Answer from the drawing. Dimensions are ordinates in mm from the lowest x, y and z of the part. Give positions to 0.01 mm unless a question says otherwise; leave off trailing zeros. Loops run counter-clockwise (first coordinate to the right, second up) from the corner with the lowest first, then second, coordinate; pieces in that order, holes last. Notation, with made-up numbers: (-0.75, 82.5) - (32.25, 82.5) arc R27 cw to (32.25, 119.5) - close; hole circle Ø2 at (47.5, 44). An arc over 180 degrees is marked (long way). One line per item, written item: value.
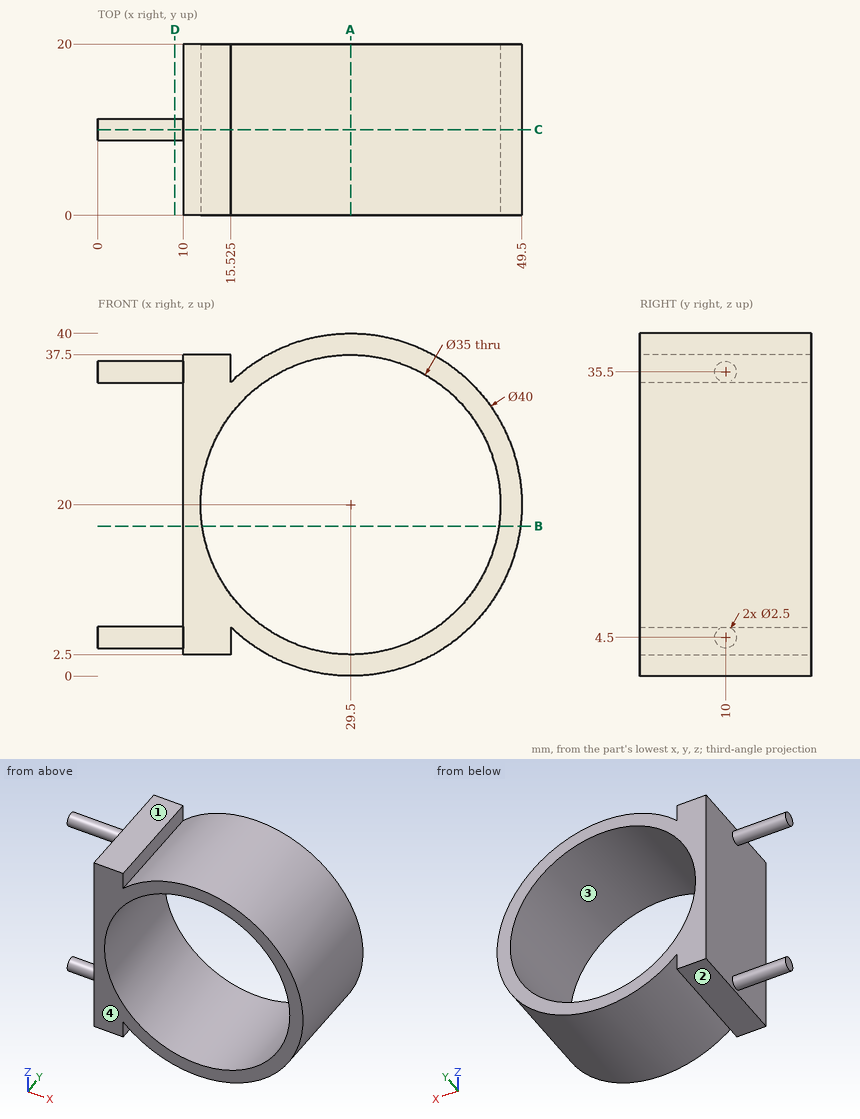
1. Flat-ended cylindrical pins translate along their axes: pin 1 Ø6 at (y, z) = (15, 11) entering from +X; pin 2 Ø3 at (x, y) = (13, 5) entering from +Z; pin 3 Ø2.5 at (y, z) = (5.5, 35.5) entering from +X; pin 4 Ø21 at (x, z) = (29.5, 20) entering from +Y. Find the tip coordinate at first contact, or state that the pin passes through.
Output:
pin 1: stops at x = 48.58
pin 2: stops at z = 37.5
pin 3: stops at x = 43.53
pin 4: passes through
2. Section A-A (x = 29.5) is taken. Write down the section's boundary in (y, z).
Output:
outline: (0, 0) - (20, 0) - (20, 2.5) - (0, 2.5) - close; (0, 37.5) - (20, 37.5) - (20, 40) - (0, 40) - close
3. Section B-B (z = 17.5) is taken. Write down the section's boundary in (x, y).
Output:
outline: (10, 0) - (12.18, 0) - (12.18, 20) - (10, 20) - close; (46.82, 0) - (49.34, 0) - (49.34, 20) - (46.82, 20) - close
4. Section D-D (x = 9) is taken. Write down the section's boundary in (y, z), and give its area (3 significant figures).
Output:
outline: circle Ø2.5 at (10, 4.5); circle Ø2.5 at (10, 35.5)
area: 9.82 mm²
5. Find the intervals of material crossed by line 1 along Z through (x, y) = (29.5, 5.75); line 2 along X through (y, z) = (11.5, 26); line 3 along Z through (x, y) = (11.5, 10), in increasing order.
Output:
line 1: z = 0 to 2.5, 37.5 to 40
line 2: x = 10 to 13.06, 45.94 to 48.58
line 3: z = 2.5 to 37.5
6. The mould has two halves that part along Z. Classify the marked faces 1, 2, 3 and 4: released by +Z, released by -Z, zero draft, split by the parting line, or undercut.
Output:
face 1: released by +Z
face 2: released by -Z
face 3: undercut
face 4: zero draft
7. Section C-C (y = 10) is taken. Write down the section's boundary in (x, z) (3 decimals), and give its area (3 significant figures).
Output:
outline: (0, 3.25) - (10, 3.25) - (10, 2.5) - (15.525, 2.5) - (15.525, 5.693) arc R20 ccw (long way) to (15.525, 34.307) - (15.525, 37.5) - (10, 37.5) - (10, 36.75) - (0, 36.75) - (0, 34.25) - (10, 34.25) - (10, 5.75) - (0, 5.75) - close; hole circle Ø35 at (29.5, 20)
area: 419 mm²
